For this review, take the finished solid that the model builds, in its own axes (mm). A direction names the side the tool comes from. Give positions to 0.01 mm unless a question says otherwise; leave off trailing zeros. Order: outer loops, then holes, each group sorted by start corner. A loop starts at its lowest first (then second) coordinate and runs counter-clockwise, first axis right, second up.
Item 1: Machinability: for faces 1 (the cylindrical face through (-0.69, 3.1, 22.05)), 2 (the cylindrical face through (-14.274, -0.628, 1.738)), which of the approach directions +Z, -Z, +X, -X, +Y, -Y give a long, thin tool a straight path to every point of the face, cutting with its end or side? Answer none if there is none.
Item 2: For P1, Ø10, axis at y = -0.5, z = 31, coming from the +X side (3 decimals); P2, Ø6, axis at y = 1, z = 26.5, coming from the -X side (3 decimals); P3, Ø6, axis at x = 1.5, z = 8.5, coming from the +Y side, all flat-tipped, find the tip position at first contact; note any pin that passes through.
Item 3: For probe 1 along Z at (x, y) = (-5.5, -1.25) (3 decimals); probe 2 along X at (y, z) = (2, 10); probe 3 along Z at (x, y) = (-9, -6.5), list the stretches that pass through material, from the lowest coordinate up.
Item 4: Consider section C-C (z = 8.5). Give the boundary of the cut face in (x, y) (1 decimal).
Item 5: Consider section A-A (x = 0). Give the boundary of the cut face in (y, z) (1 decimal).
Autodesk Inventor part; units mm, degrees
ref_plane "YZ Plane" through (0, 0, 0) normal (1, 0, 0) x (0, 1, 0)
ref_plane "XZ Plane" through (0, 0, 0) normal (0, 1, 0) x (-1, 0, 0)
ref_plane "XY Plane" through (0, 0, 0) normal (0, 0, 1) x (1, 0, 0)
sketch "Sketch1" plane through (0, 0, 0) normal (0, 0, 1) x (1, 0, 0)
  circle A0 centre (0, 0) radius 14.2875
  dimension "d0" = 28.575
extrude "Extrusion1" add sketch "Sketch1" along normal blind 9.525
sketch "Sketch2" plane through (0, 0, 9.525) normal (0, 0, 1) x (1, 0, 0)
  circle A0 centre (0, 0) radius 14.2875
  circle A1 centre (0, 0) radius 3.175
  dimension "d4" = 6.35
extrude "Extrusion2" add sketch "Sketch2" along normal blind 25.4 contours A1
chamfer "Chamfer1" distance 6 angle 45 1 edges at (-14.2875, 0, 9.525)
thread "Thread1"
properties part number "23015T82"
Resolved:
1. face 1: +Z
1. face 2: +Z, -Z
2. P1: stops at x = 3.175
2. P2: stops at x = -3.175
2. P3: stops at y = 12.24
3. probe 1: z = 0 to 9.525
3. probe 2: x = -2.47 to 2.47
3. probe 3: z = 0 to 6.71
4. outline: circle Ø18.6 at (0, 0)
5. outline: (-14.3, 0) - (14.3, 0) - (14.3, 3.5) - (8.3, 9.5) - (3.2, 9.5) - (3.2, 34.9) - (-3.2, 34.9) - (-3.2, 9.5) - (-8.3, 9.5) - (-14.3, 3.5) - close
